from build123d import *

# Parameters (mm, degrees)
SKETCH_1_W               = 20
SKETCH_1_H               = 20
SKETCH_1_R               = 2
SKETCH_1_R_2             = 2.15
EXTRUDE_1_DEPTH          = 80
CUT_EXTRUDE_1_REACH      = 83.24
PATTERN_CIRCULAR_1_COUNT = 4
FILLET_1_R               = 0.3
SKETCH_3_R               = 2.5
CUT_EXTRUDE_2_DEPTH      = 84.066238629


with BuildPart() as part:
    # Sketch 1 → Extrude 1 (new body)
    with BuildSketch(Plane.XY):
        Rectangle(SKETCH_1_W, SKETCH_1_H)
        with Locations((-7, 7)):
            Circle(SKETCH_1_R, mode=Mode.SUBTRACT)
        with Locations((-7, -7)):
            Circle(SKETCH_1_R, mode=Mode.SUBTRACT)
        Circle(SKETCH_1_R_2, mode=Mode.SUBTRACT)
        with Locations((7, 7)):
            Circle(SKETCH_1_R, mode=Mode.SUBTRACT)
        with Locations((7, -7)):
            Circle(SKETCH_1_R, mode=Mode.SUBTRACT)
    extrude(amount=EXTRUDE_1_DEPTH)

    # Sketch 1_3 → Cut-Extrude 1 (cut, up to next)
    with BuildSketch(Plane.XY, mode=Mode.PRIVATE) as cut_extrude_1_sk1:
        with BuildLine():
            Line((-8.5, 2.65), (-10, 2.65))
            Line((-10, 2.65), (-10, -2.65))
            Line((-10, -2.65), (-8.5, -2.65))
            Line((-8.5, -2.65), (-8.5, -4.15))
            Line((-8.5, -4.15), (-4.503166667, -4.15))
            ThreePointArc((-4.503166667, -4.15), (-3.3, 0), (-4.503166667, 4.15))
            Line((-4.503166667, 4.15), (-8.5, 4.15))
            Line((-8.5, 4.15), (-8.5, 2.65))
        make_face()
    cut_extrude_1_tool1 = extrude(cut_extrude_1_sk1.sketch, amount=CUT_EXTRUDE_1_REACH, mode=Mode.PRIVATE) & part.part
    cut_extrude_1 = cut_extrude_1_tool1.solids().sort_by_distance((-6.606913, 0, 0))[0]
    add(cut_extrude_1, mode=Mode.SUBTRACT)

    # Pattern Circular 1: Cut-Extrude 1 ×4 about axis
    pattern_circular_1_axis = Axis((0, 0, 0), (0, 0, 1))
    for i in range(1, PATTERN_CIRCULAR_1_COUNT):
        add(cut_extrude_1.rotate(pattern_circular_1_axis, i * 360 / PATTERN_CIRCULAR_1_COUNT), mode=Mode.SUBTRACT)

    # Fillet 1
    fillet_1_edges = [part.edges().sort_by_distance(p)[0] for p in [
        (-10, -10, 40),
        (10, -10, 40),
        (10, 10, 40),
        (-10, 10, 40),
    ]]
    fillet(fillet_1_edges, radius=FILLET_1_R)

    # Sketch 3 → Cut-Extrude 2 (cut, through all)
    with BuildSketch(Plane.XZ.offset(10)):
        with Locations(Location((0, 69, 0), (0, 0, 270))):
            Circle(SKETCH_3_R)
        with Locations(Location((0, 11, 0), (0, 0, 270))):
            Circle(SKETCH_3_R)
    extrude(amount=-CUT_EXTRUDE_2_DEPTH, mode=Mode.SUBTRACT)


solid = part.part
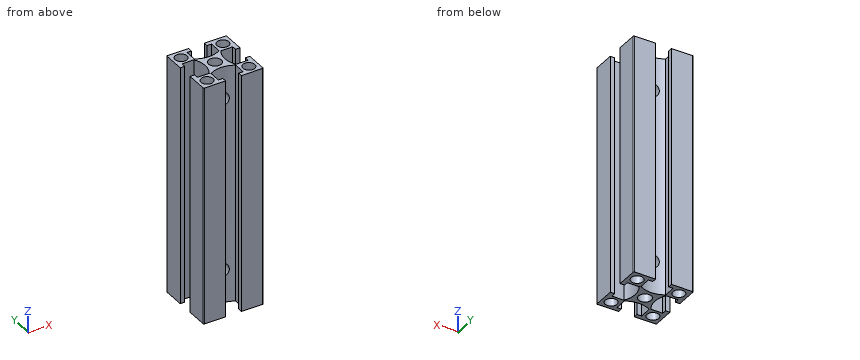
Geometry check sheet. Reference: the model listing, model coordinates, mm. Round coordinates to 2 decimals unless told otherwise and drop trailing zeros. Write each loop counter-clockwise with the first axis right and the second up, starting at its lowest first coordinate (ties: lowest second). Pieces come first, ordered by that corner, then holes. Notation, with made-up numbers: (51.25, 79) - (55.25, 79) arc R20 ccw to (55.25, 85) - close; hole circle Ø10 at (30.25, 87.25). An arc over 180 degrees is marked (long way). One line per item, written item: value.
1. Depth check by flat-ended pin: pin 1 Ø3.5 at (x, y) = (-7, 7) entering from +Z. Enter the tip coordinate at first touch or a pass-through.
The answers:
pin 1: passes through
2. Cross-section at D-D on z = 11. Give the number of separate pieces and of enclosed holes in the cut face, and give its area (3 significant figures).
The answers:
separate pieces: 2
enclosed holes: 4
area: 124 mm^2
3. Scan lines: L1, parallel to Y at x = 7, z = 50.5; L2, parallel to Y at x = 0, z = 6.25. Record each from-to range of solid material in increasing order.
The answers:
L1: y = -10 to -9, -5 to -4.15, 4.15 to 5, 9 to 10
L2: y = -3.3 to -2.15, 2.15 to 3.3
4. Cross-section at A-A on y = 7. Record the boundary of the cut face in (x, z).
The answers:
outline: (-10, 0) - (-9, 0) - (-9, 80) - (-10, 80) - close; (-5, 0) - (-4.15, 0) - (-4.15, 80) - (-5, 80) - close; (4.15, 0) - (5, 0) - (5, 80) - (4.15, 80) - close; (9, 0) - (10, 0) - (10, 80) - (9, 80) - close
5. Cross-section at C-C on y = 0. Record the boundary of the cut face in (x, z), and give its area (3 significant figures).
The answers:
outline: (-3.3, 0) - (-2.15, 0) - (-2.15, 9.72) arc R2.5 cw to (-2.15, 12.28) - (-2.15, 67.72) arc R2.5 cw to (-2.15, 70.28) - (-2.15, 80) - (-3.3, 80) - close; (2.15, 0) - (3.3, 0) - (3.3, 80) - (2.15, 80) - (2.15, 70.28) arc R2.5 cw to (2.15, 67.72) - (2.15, 12.28) arc R2.5 cw to (2.15, 9.72) - close
area: 182 mm^2
6. Cross-section at B-B on x = 0. Record the boundary of the cut face in (y, z).
The answers:
outline: (-3.3, 0) - (-2.15, 0) - (-2.15, 8.5) - (-3.3, 8.5) - close; (-3.3, 13.5) - (-2.15, 13.5) - (-2.15, 66.5) - (-3.3, 66.5) - close; (-3.3, 71.5) - (-2.15, 71.5) - (-2.15, 80) - (-3.3, 80) - close; (2.15, 0) - (3.3, 0) - (3.3, 8.5) - (2.15, 8.5) - close; (2.15, 13.5) - (3.3, 13.5) - (3.3, 66.5) - (2.15, 66.5) - close; (2.15, 71.5) - (3.3, 71.5) - (3.3, 80) - (2.15, 80) - close
